```python
from build123d import *

# Parameters (mm, degrees)
EXTRUDE_1_DEPTH = 3.5
SKETCH_2_R      = 2.5
EXTRUDE_2_DEPTH = 13


with BuildPart() as part:
    # ｽｹｯﾁ1 → ﾎﾞｽ - 押し出し1 (new body)
    with BuildSketch(Plane.XY):
        Polygon((-2.979795067, -3.529044445), (1.566344606, -4.345100448), (4.546139674, -0.816056004), (2.979795067, 3.529044445), (-1.566344606, 4.345100448), (-4.546139674, 0.816056004), align=None)
    extrude(amount=EXTRUDE_1_DEPTH)

    # ｽｹｯﾁ2 → ﾎﾞｽ - 押し出し2 (add)
    with BuildSketch(Plane.XY.offset(3.5)):
        with Locations(Location((0, 0, 0), (0, 0, 180))):
            Circle(SKETCH_2_R)
    extrude(amount=EXTRUDE_2_DEPTH)


solid = part.part
```
Verification items for the finished model (mm, model axes). A direction names the side the tool comes from. Give positions to 0.01 mm unless a question says otherwise; leave off trailing zeros. Order: outer loops, then holes, each group sorted by start corner. A loop starts at its lowest first (then second) coordinate and runs counter-clockwise, first axis right, second up. Notation, with made-up numbers: M -20.75,80 L 5.25,80 A27 cw 5.25,115 Z; hole C 81,48 d6. An arc over 180 degrees is marked long. Answer in a Markdown table with one row per item. Add a question column.
Item 1: Section check D-D, the plane z = 5.5. Enter the section's corners in (x, y).
Item 2: Section check B-B, the plane y = -0.5. Enter the section's corners in (x, z).
Item 3: Scan lines: probe 1 along Z at (x, y) = (-2.25, 2.5); probe 2 along X at (y, z) = (0.5, 8); probe 3 along Y at (x, z) = (-0.75, 1.25). Record each from-to range of solid material in increasing order. Write a range as from..to.
Item 4: Tool access check on faces 1 (the flat face through (3.035, -2.605, 1.726)), 2 (the flat face through (2, -2, 3.5)). Record the directions out of +Z, -Z, +X, -X, +Y, -Y that give a thin tool (end or side, any length) a straight path to the whole face; none if there is none.
Item 5: Section check A-A, the plane z = 3. Enter the section's corners in (x, y).
Item 6: Section check C-C, the plane x = 2. Enter the section's corners in (y, z), and give its area (3 significant figures).
Item 7: Gauge pin test, flat ends, axial feed: pin 1 (2 mm diameter, centred on x = 1.5, z = 8, fed in from -Y); pin 2 (2 mm diameter, centred on y = -0.5, z = 8.5, fed in from -X). Record the tip position at first contact, or that the pin passes through.
Filled sheet:
| question | item | result |
|---|---|---|
| 1 | outline | C 0,0 d5 |
| 2 | outline | M -4.07,0 L 4.43,0 L 4.43,3.5 L 2.45,3.5 L 2.45,16.5 L -2.45,16.5 L -2.45,3.5 L -4.07,3.5 Z |
| 3 | probe 1 | z = 0..3.5 |
| 3 | probe 2 | x = -2.45..2.45 |
| 3 | probe 3 | y = -3.93..4.2 |
| 4 | face 1 | +Z, -Z, +X, -Y |
| 4 | face 2 | +Z |
| 5 | outline | M -4.55,0.82 L -2.98,-3.53 L 1.57,-4.35 L 4.55,-0.82 L 2.98,3.53 L -1.57,4.35 Z |
| 6 | outline | M -3.83,0 L 3.7,0 L 3.7,3.5 L 1.5,3.5 L 1.5,16.5 L -1.5,16.5 L -1.5,3.5 L -3.83,3.5 Z |
| 6 | area | 65.4 mm^2 |
| 7 | pin 1 | stops at y = -2.45 |
| 7 | pin 2 | stops at x = -2.5 |
